Model file for the job. Use its own axes, mm. A direction names the side the tool comes from. Round coordinates to 2 decimals unless told otherwise and drop trailing zeros. Order: outer loops, then holes, each group sorted by start corner. A loop starts at its lowest first (then second) coordinate and runs counter-clockwise, first axis right, second up. Notation, with made-up numbers: (-1.5, 29) - (22.5, 29) arc R13 cw to (22.5, 45) - close; hole circle Ø2 at (76, 17.25). An arc over 180 degrees is marked (long way). Write item = value, one per line.
```python
from build123d import *

# Parameters (mm, degrees)
F1_DEPTH = 2.54
F2_DEPTH = 2.54
F3_DEPTH = 5.08
F5_DEPTH = 3


with BuildPart() as f1:
    # F0 (on Top) → F1 (new body)
    with BuildSketch(Plane.XY):
        with BuildLine():
            Line((0, -15), (0, 15))
            ThreePointArc((0, 15), (-15, 0), (0, -15))
        make_face()
    extrude(amount=F1_DEPTH)

    # F0 (on Top) + F1_face (on face) → F2 (join)
    with BuildSketch(Plane.XY):
        with BuildLine():
            Line((0, 15), (0, 15.15))
            ThreePointArc((0, 15.15), (-15.15, 0), (0, -15.15))
            Line((0, -15.15), (0, -15))
            ThreePointArc((0, -15), (-15, 0), (0, 15))
        make_face()
    with BuildSketch(Plane(origin=(-6.3661977237, 0, 2.54), x_dir=(1, 0, 0), z_dir=(0, 0, 1))):
        with BuildLine():
            ThreePointArc((6.3661977237, 15), (-8.6338022763, 0), (6.3661977237, -15))
            Line((6.3661977237, -15), (6.3661977237, 15))
        make_face()
    extrude(amount=F2_DEPTH)

    # F0 (on Top) → F3 (join)
    with BuildSketch(Plane.XY):
        with BuildLine():
            Line((0, 15.15), (0, 15.5))
            ThreePointArc((0, 15.5), (-15.5, 0), (0, -15.5))
            Line((0, -15.5), (0, -15.15))
            ThreePointArc((0, -15.15), (-15.15, 0), (0, 15.15))
        make_face()
    extrude(amount=F3_DEPTH)

    # F4 (on Right) → F5 (join)
    with BuildSketch(Plane.YZ):
        Polygon((15.5500713736, -11.4404093474), (27.990128845, -11.4404093474), (27.990128845, 43.2069823146), (-70.4196095467, 43.2069823146), (-70.4196095467, -11.4404093474), align=None)
    extrude(amount=-F5_DEPTH)


solid = f1.part
```
1) Cut at D-D (y = -27). Write the cut outline in (x, z).
Conclusion:
outline = (-3, -11.44) - (0, -11.44) - (0, 43.21) - (-3, 43.21) - close
2) Cut at C-C (z = 10.5). Write the cut outline in (x, y), and give its area (3 significant figures).
Conclusion:
outline = (-3, -70.42) - (0, -70.42) - (0, 27.99) - (-3, 27.99) - close
area = 295 mm^2
3) Flat gauge pins, fed straight in: pin 1 Ø6 at (x, y) = (-6.5, -6.5) entering from +Z; pin 2 Ø1 at (y, z) = (-2.5, 3.5) entering from -X; pin 3 Ø5 at (x, z) = (-5, 37) entering from +Y; pin 4 Ø4 at (y, z) = (-4.5, 17.5) entering from -X. Where does each tip first touch, or does it go through?
Conclusion:
pin_1 = 5.08
pin_2 = -15.37
pin_3 = 27.99
pin_4 = -3
4) Cut at A-A (y = -4). Write the cut outline in (x, z).
Conclusion:
outline = (-14.97, 0) - (-3, 0) - (-3, -11.44) - (0, -11.44) - (0, 43.21) - (-3, 43.21) - (-3, 5.08) - (-14.46, 5.08) - (-14.46, 2.54) - (-14.61, 2.54) - (-14.61, 5.08) - (-14.97, 5.08) - close
5) Wall check: line 1 along Y through (x, z) = (-8, 4); line 2 along X through (y, z) = (-47.5, 20); line 3 along Z through (x, y) = (-7, -5). Give the ranges that are in metal, low to high.
Conclusion:
line_1 = -13.28 to -12.87, -12.69 to 12.69, 12.87 to 13.28
line_2 = -3 to 0
line_3 = 0 to 5.08
6) Cut at B-B (x = -4.5). Write the cut outline in (y, z).
Conclusion:
outline = (-14.83, 0) - (14.83, 0) - (14.83, 5.08) - (14.47, 5.08) - (14.47, 2.54) - (14.31, 2.54) - (14.31, 5.08) - (-14.31, 5.08) - (-14.31, 2.54) - (-14.47, 2.54) - (-14.47, 5.08) - (-14.83, 5.08) - close
7) Mould opens along Y. For faces 4 (the face through (-15.3, 0.1, 5.08)), 5 (the face through (-1, -70.42, 16)), 6 (the face through (-14.997, 0.288, 3.792)) say: +Y half, -Y half, draft (parallel to the pull), parting line (faces both ways), or undercut.
Conclusion:
face_4 = draft
face_5 = -Y half
face_6 = undercut
8) 3-axis set-ups, long thin cutter, end or side, ignore diameter. For faces 1 (the face through (-8, 0, 5.08)), 2 (the face through (-1, -21, 43.207)), 3 (the face through (-8, 0, 0)): which of +Z, -Z, +X, -X, +Y, -Y reach the whole face in a straight line?
Conclusion:
face_1 = +Z, -X, +Y, -Y
face_2 = +Z, +X, -X, +Y, -Y
face_3 = -Z, -X, +Y, -Y
